from build123d import *

# Parameters (mm, degrees)
PAD001_DEPTH    = 5
SKETCH006_R     = 2
POCKET003_DEPTH = 20
SKETCH008_R     = 3
PAD002_DEPTH    = 5
SKETCH007_R     = 1.1
SKETCH007_W     = 20
SKETCH007_H     = 9
POCKET004_DEPTH = 20


with BuildPart() as part:
    # Sketch005 → Pad001 (new body)
    with BuildSketch(Plane.XY):
        with BuildLine():
            ThreePointArc((-35, 25), (-38.535534, 23.535534), (-40, 20))
            Line((-40, -20), (-40, 20))
            ThreePointArc((-40, -20), (-38.535534, -23.535534), (-35, -25))
            Line((35, -25), (-35, -25))
            ThreePointArc((35, -25), (38.535534, -23.535534), (40, -20))
            Line((40, 20), (40, -20))
            ThreePointArc((40, 20), (38.535534, 23.535534), (35, 25))
            Line((-35, 25), (35, 25))
        make_face()
    extrude(amount=PAD001_DEPTH)

    # Sketch006 (on Face10 of Pad001) → Pocket003 (cut)
    with BuildSketch(Plane.XY.offset(5)):
        with Locations((-35, 20)):
            Circle(SKETCH006_R)
        with Locations((35, 20)):
            Circle(SKETCH006_R)
        with Locations((35, -20)):
            Circle(SKETCH006_R)
        with Locations((-35, -20)):
            Circle(SKETCH006_R)
    extrude(amount=-POCKET003_DEPTH, mode=Mode.SUBTRACT)

    # Sketch008 → Pad002 (join)
    with BuildSketch(Plane(origin=(0, 0, 0), x_dir=(1, 0, 0), z_dir=(0, 0, -1))):
        with Locations((-13, 5.5)):
            Circle(SKETCH008_R)
        with Locations((13, 5.5)):
            Circle(SKETCH008_R)
        with Locations((13, -5.5)):
            Circle(SKETCH008_R)
        with Locations((-13, -5.5)):
            Circle(SKETCH008_R)
    extrude(amount=PAD002_DEPTH)

    # Sketch007 (on Face5 of Pocket003) → Pocket004 (cut)
    with BuildSketch(Plane.XY.offset(5)):
        with Locations((-13, 5.5)):
            Circle(SKETCH007_R)
        with Locations((13, 5.5)):
            Circle(SKETCH007_R)
        with Locations((13, -5.5)):
            Circle(SKETCH007_R)
        with Locations((-13, -5.5)):
            Circle(SKETCH007_R)
        Rectangle(SKETCH007_W, SKETCH007_H)
    extrude(amount=-POCKET004_DEPTH, mode=Mode.SUBTRACT)


solid = part.part
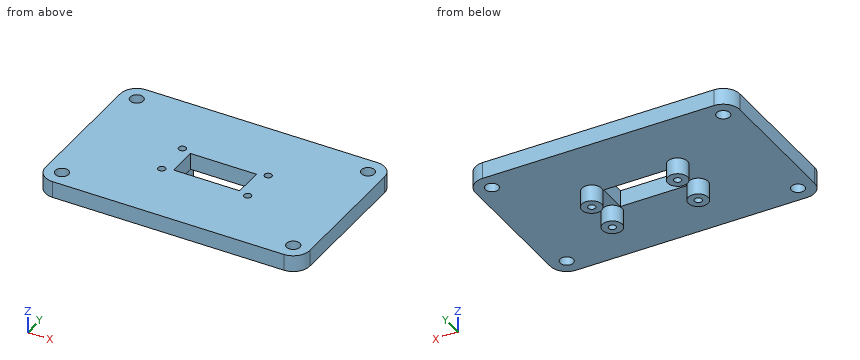
Can you work these out from the model? Positions are in its coordinate system, mm. Coordinates: 2 decimals unless noted, no trailing zeros. Write each loop counter-clockwise with the first axis right and the second up, starting at its lowest first coordinate (ties: lowest second). Pieces come first, ordered by that corner, then holes. Notation, with made-up numbers: M 7.25,-19 L 38.25,-19 A36 cw 38.25,15 Z; hole C 47,-35.5 d4. An arc over 180 degrees is marked long. Use one line per item in the form item = value.
Q1. If we section it at D-D (x = -13): Write out the boundary of the cut face in (y, z), then the cut area to 3 significant figures.
Model answer:
outline = M -25,0 L -8.5,0 L -8.5,-5 L -6.6,-5 L -6.6,5 L -25,5 Z; M -4.4,-5 L -2.5,-5 L -2.5,0 L 2.5,0 L 2.5,-5 L 4.4,-5 L 4.4,5 L -4.4,5 Z; M 6.6,-5 L 8.5,-5 L 8.5,0 L 25,0 L 25,5 L 6.6,5 Z
area = 266 mm^2
Q2. If we section it at C-C (y = 5.5): Write out the boundary of the cut face in (x, z).
Model answer:
outline = M -40,0 L -16,0 L -16,-5 L -14.1,-5 L -14.1,5 L -40,5 Z; M -11.9,-5 L -10,-5 L -10,0 L 10,0 L 10,-5 L 11.9,-5 L 11.9,5 L -11.9,5 Z; M 14.1,-5 L 16,-5 L 16,0 L 40,0 L 40,5 L 14.1,5 Z
Q3. If we section it at B-B (z = 1.75): State how many separate pieces and enclosed holes the cut face has, then the cut area to 3 significant figures.
Model answer:
separate_pieces = 1
enclosed_holes = 9
area = 3,730 mm^2
Q4. I need wall thicknesses on line 1 along Y through (x, z) = (-13, -1.25); line 2 along Y through (x, z) = (-35, 2.1); line 3 along Y through (x, z) = (-13, 0.5). Which ranges of each line are inside material? Lowest first, please. Write a range as from..to.
Model answer:
line_1 = -8.5..-6.6, -4.4..-2.5, 2.5..4.4, 6.6..8.5
line_2 = -25..-22, -18..18, 22..25
line_3 = -25..-6.6, -4.4..4.4, 6.6..25
Q5. If we section it at A-A (x = 8): Write out the boundary of the cut face in (y, z), then the cut area to 3 significant figures.
Model answer:
outline = M -25,0 L -4.5,0 L -4.5,5 L -25,5 Z; M 4.5,0 L 25,0 L 25,5 L 4.5,5 Z
area = 205 mm^2
Q6. For P1, Ø6.5, axis at x = -35, y = -20, coming from the -Z side, with a flat end and sliding along its axis, tell me the tip position at first contact or that it passes through.
Model answer:
P1 = 0
